Here's how the part is built. I have some questions about the finished solid (model axes, mm). A direction names the side the tool comes from. Round coordinates to 2 decimals unless told otherwise and drop trailing zeros. Order: outer loops, then holes, each group sorted by start corner. A loop starts at its lowest first (then second) coordinate and runs counter-clockwise, first axis right, second up. Notation, with made-up numbers: M 80,56.25 L 106,56.25 A24 cw 106,82.25 Z; hole C 44.5,57.25 d5. An arc over 180 degrees is marked long. Write item = value, one per line. Start each with the question number.
Item 1: I want a section at C-C, the plane y = 0.45. List the corners of the cut face in (x, z) for me.
Item 2: Please list where these lines run through material, in increasing order: L1, parallel to X at y = 0.8, z = 0; L2, parallel to X at y = 1.3, z = 0; L3, parallel to X at y = 0.5, z = 2.75.
Item 3: For faces 1 (the face through (-1.5, 1.35, -0.07)), 2 (the face through (-5.25, 0.51, -0.03)), which set-ups out of +Z, -Z, +X, -X, +Y, -Y let a thin tool reach every point of the face, with its end or its side?
Item 4: I'm going to push flat-ended pins straight in: P1, Ø5, axis at x = 4, z = -3, coming from the +Y side; P2, Ø1.2, axis at x = 4.5, z = 0, coming from the -Y side. Where does each tip first touch, or does it pass through?
Item 5: I want a section at D-D, the plane x = 0. List the corners of the cut face in (y, z) for me.
Item 6: We'd pull the mould along X, two halves only. Please class faces 3 (the face through (-5.699, 0.507, 4.715)), 4 (the face through (6, 0.5, 0.1)), 5 (the face through (3.905, 0.507, 0.456)): pulls with the +X half, pulls with the -X half, needs draft (parallel to the pull), parting line crosses it, or undercut.
Item 7: I want a section at B-B, the plane x = -4.5. State how many separate pieces and enclosed holes the cut face has, plus the area to 3 significant figures.
```python
from build123d import *

# Parameters (mm, degrees)
SALIENTE_EXTRUIR1_DEPTH = 1
REDONDEO1_R             = 1
CROQUIS2_R              = 1.5
CORTAR_EXTRUIR3_DEPTH   = 0.01
CROQUIS5_R              = 0.75
CORTAR_EXTRUIR5_DEPTH   = 1.1
CROQUIS6_R              = 0.75
CROQUIS6_R_2            = 0.5
CORTAR_EXTRUIR6_DEPTH   = 1.1
CROQUIS7_R              = 2
SALIENTE_EXTRUIR2_DEPTH = 0.7
CROQUIS8_R              = 1.5
CORTAR_EXTRUIR7_DEPTH   = 0.7
CROQUIS9_R              = 0.5
CORTAR_EXTRUIR9_DEPTH   = 8


with BuildPart() as part:
    # Croquis1 → Saliente-Extruir1 (new body)
    with BuildSketch(Plane(origin=(0, 0, 0), x_dir=(1, 0, 0), z_dir=(0, 1, 0))):
        Polygon((-6, 5), (6, 5), (6, 0.5), (6, -5), (1.5, -5), (-6, -5), align=None)
    extrude(amount=SALIENTE_EXTRUIR1_DEPTH)

    # Redondeo1
    redondeo1_edges = [part.edges().sort_by_distance(p)[0] for p in [
        (-6, 0.5, -5),
        (6, 0.5, -5),
        (6, 0.5, 5),
        (-6, 0.5, 5),
    ]]
    fillet(redondeo1_edges, radius=REDONDEO1_R)

    # Croquis2 → Cortar-Extruir3 (cut)
    with BuildSketch(Plane(origin=(0, 1, 0), x_dir=(1, 0, 0), z_dir=(0, 1, 0))):
        with Locations((4, 3)):
            Circle(CROQUIS2_R)
        with Locations((-4, -3)):
            Circle(CROQUIS2_R)
    extrude(amount=-CORTAR_EXTRUIR3_DEPTH, mode=Mode.SUBTRACT)

    # Croquis5 → Cortar-Extruir5 (cut)
    with BuildSketch(Plane(origin=(0, 0.99, 0), x_dir=(1, 0, 0), z_dir=(0, 1, 0))):
        with Locations((4, 3)):
            Circle(CROQUIS5_R)
        with Locations((-4, -3)):
            Circle(CROQUIS5_R)
    extrude(amount=-CORTAR_EXTRUIR5_DEPTH, mode=Mode.SUBTRACT)

    # Croquis6 → Cortar-Extruir6 (cut)
    with BuildSketch(Plane(origin=(0, 1, 0), x_dir=(1, 0, 0), z_dir=(0, 1, 0))):
        with Locations((4.5, 0)):
            Circle(CROQUIS6_R)
        with Locations((-4.5, 0)):
            Circle(CROQUIS6_R)
        with Locations((3.36, -2.36)):
            Circle(CROQUIS6_R_2)
        with Locations((-3.36, 2.36)):
            Circle(CROQUIS6_R_2)
    extrude(amount=-CORTAR_EXTRUIR6_DEPTH, mode=Mode.SUBTRACT)

    # Croquis7 → Saliente-Extruir2 (add)
    with BuildSketch(Plane(origin=(0, 1, 0), x_dir=(1, 0, 0), z_dir=(0, 1, 0))):
        Circle(CROQUIS7_R)
    extrude(amount=SALIENTE_EXTRUIR2_DEPTH)

    # Croquis8 → Cortar-Extruir7 (cut)
    with BuildSketch(Plane(origin=(0, 1.7, 0), x_dir=(1, 0, 0), z_dir=(0, 1, 0))):
        Circle(CROQUIS8_R)
    extrude(amount=-CORTAR_EXTRUIR7_DEPTH, mode=Mode.SUBTRACT)

    # Croquis9 → Cortar-Extruir9 (cut)
    with BuildSketch(Plane(origin=(0, 1, 0), x_dir=(1, 0, 0), z_dir=(0, 1, 0))):
        Circle(CROQUIS9_R)
    extrude(amount=-CORTAR_EXTRUIR9_DEPTH, mode=Mode.SUBTRACT)


solid = part.part
```
Filled in:
q1.outline = M -6,-4 A1 ccw -5,-5 L 5,-5 A1 ccw 6,-4 L 6,4 A1 ccw 5,5 L -5,5 A1 ccw -6,4 Z; hole C -4.5,0 d1.5; hole C -4,3 d1.5; hole C -3.36,-2.36 d1; hole C 0,0 d1; hole C 3.36,2.36 d1; hole C 4,-3 d1.5; hole C 4.5,0 d1.5
q2.L1 = -6 to -5.25, -3.75 to -0.5, 0.5 to 3.75, 5.25 to 6
q2.L2 = -2 to -1.5, 1.5 to 2
q2.L3 = -6 to -4.71, -3.29 to 3.05, 3.67 to 6
q3.face_1 = +Y
q3.face_2 = +Y, -Y
q4.P1 = 1
q4.P2 = through
q5.outline = M 0,-5 L 1,-5 L 1,-2 L 1.7,-2 L 1.7,-1.5 L 1,-1.5 L 1,-0.5 L 0,-0.5 Z; M 0,0.5 L 1,0.5 L 1,1.5 L 1.7,1.5 L 1.7,2 L 1,2 L 1,5 L 0,5 Z
q6.face_3 = pulls with the -X half
q6.face_4 = pulls with the +X half
q6.face_5 = undercut
q7.separate_pieces = 3
q7.enclosed_holes = 0
q7.area = 7.36 mm^2
